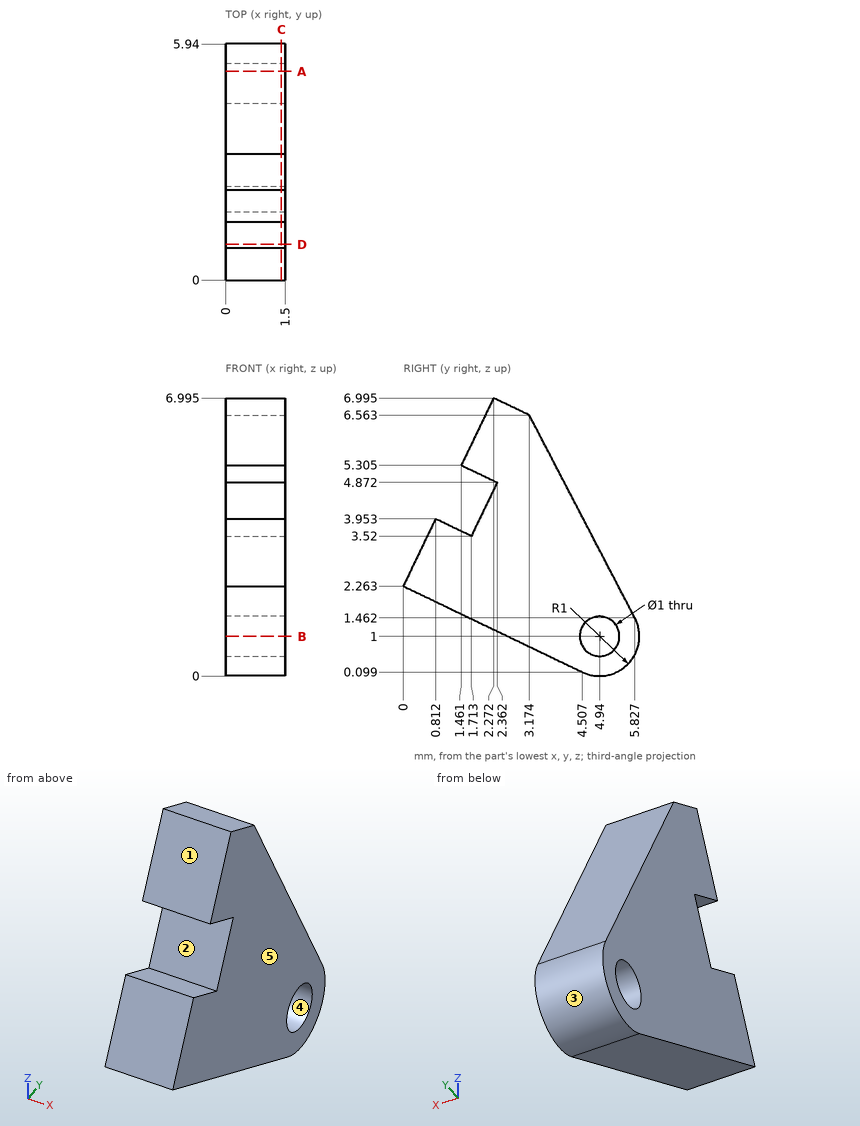
Design review of the part shown in the three views and the two pictorial views. Dimensions are in mm from the part's minimum x, y and z. A direction names the side the tool comes from. Round coordinates to 2 decimals unless told otherwise and drop trailing zeros. Write each loop counter-clockwise with the first axis right and the second up, starting at its lowest first coordinate (ties: lowest second). Pieces come first, ordered by that corner, then holes.
Item 1: Consider section B-B on z = 1. Give the boundary of the cut face in (x, y).
Item 2: Draft analysis for pull direction Y (two halves, no side actions). For the marked faces 3, 4 and 5, state which applies: released by +Y, released by -Y, zero draft, split by the parting line, or undercut.
Item 3: Wall thickness on L1, parallel to Y at x = 1, z = 3.75 (1 decimal); L2, parallel to Z at x = 0.1, y = 5.05 (1 decimal); L3, parallel to Y at x = 0.9, z = 1.25 (1 decimal): over which ranges is each line inside the solid? List them lowest first.
Item 4: Consider section D-D on y = 0.9. Give the boundary of the cut face in (x, z).
Item 5: Consider section A-A on y = 5.25. Give the boundary of the cut face in (x, z).
Item 6: Consider section C-C on x = 1.4. Give the boundary of the cut face in (y, z) (1 decimal), and give its area (3 significant figures).
Item 7: For the marked faces 1 and 2, list the 3-axis set-ups (+Z, -Z, +X, -X, +Y, -Y) from which the entire face can be reached by the end or side of a thin tool; tool diameter is ignored.
Check values:
1. outline: (0, 2.63) - (1.5, 2.63) - (1.5, 4.44) - (0, 4.44) - close; (0, 5.44) - (1.5, 5.44) - (1.5, 5.94) - (0, 5.94) - close
2. face 3: split by the parting line
2. face 4: undercut
2. face 5: zero draft
3. L1: y = 0.7 to 1.2, 1.8 to 4.6
3. L2: z = 0 to 0.5, 1.5 to 3
3. L3: y = 2.1 to 4.5, 5.4 to 5.9
4. outline: (0, 1.83) - (1.5, 1.83) - (1.5, 3.91) - (0, 3.91) - close
5. outline: (0, 0.05) - (1.5, 0.05) - (1.5, 0.61) - (0, 0.61) - close; (0, 1.39) - (1.5, 1.39) - (1.5, 2.57) - (0, 2.57) - close
6. outline: (0, 2.3) - (4.5, 0.1) arc R1 ccw to (5.8, 1.5) - (3.2, 6.6) - (2.3, 7) - (1.5, 5.3) - (2.4, 4.9) - (1.7, 3.5) - (0.8, 4) - close; hole circle Ø1 at (4.9, 1)
6. area: 19.6 mm2
7. face 1: +Z, +X, -X, -Y
7. face 2: +X, -X
